Source: CAD feature listing. Evaluate the final solid. Frame: model axes, mm. Round coordinates to 2 decimals unless told otherwise and drop trailing zeros. Loops run counter-clockwise (first coordinate to the right, second up) from the corner with the lowest first, then second, coordinate; pieces in that order, holes last. Notation, with made-up numbers: M 37,12 L 46,12 A8 ccw 46,23 Z; hole C 42,72.25 d5. An arc over 180 degrees is marked long. Write each question's results on one line, items separated by ' | '. Start each with the question number.
1. Contact query for flat-ended pins moving along their axis: pin 1 Ø6 at (x, z) = (29.5, 2.5) entering from -Y; pin 2 Ø2 at (y, z) = (4, 26) entering from -X; pin 3 Ø8 at (y, z) = (4, -23) entering from -X; pin 4 Ø3 at (x, y) = (17.5, 6.5) entering from -Z. Output: stop coordinate, or through.
2. Ray query, line 1 (X direction, y = 5.5, z = -28.5); line 2 (Z direction, x = 7.5, y = 13); line 3 (X direction, y = 5.75, z = 32.5). Return the intervals inside material, ascending.
3. Draft query along X for faces 1 (the cylindrical face through (34.534, 7.395, 14.383)), 2 (the cylindrical face through (37.41, 7.4, 0.07)), 3 (the cylindrical face through (-34.59, 7.4, 14.25)). Return one class per face: released by +X, released by -X, zero draft, split by the parting line, or undercut.
4. Section B-B on z = 0. Output: boundary loops of the cut face in (x, y).
5. Section A-A on x = 0. Output: boundary loops of the cut face in (y, z), and give its area (3 significant figures).
6. Section C-C on z = -21. Output: boundary loops of the cut face in (x, y).
from build123d import *

# Parameters (mm, degrees)
SKETCH1_R           = 11
BOSS_EXTRUDE1_DEPTH = 15


with BuildPart() as part:
    # Sketch1 → Boss-Extrude1 (new body)
    with BuildSketch(Plane(origin=(0, 0, 0), x_dir=(1, 0, 0), z_dir=(0, 1, 0))):
        with BuildLine():
            ThreePointArc((40.667554182, -3.397048659), (37.40918895, 0), (40.667554182, 3.397048659))
            ThreePointArc((40.667554182, 3.397048659), (40.61268155, 4), (40.548869848, 4.602070919))
            ThreePointArc((40.548869848, 4.602070919), (36.690381874, 7.298170719), (39.223407215, 11.265621563))
            ThreePointArc((39.223407215, 11.265621563), (39.051958974, 11.846282243), (38.871915187, 12.424335493))
            ThreePointArc((38.871915187, 12.424335493), (34.561583998, 14.315876829), (36.271926705, 18.701262947))
            ThreePointArc((36.271926705, 18.701262947), (35.990491515, 19.237318503), (35.701134624, 19.769139821))
            ThreePointArc((35.701134624, 19.769139821), (31.104603832, 20.783431822), (31.926536394, 25.418225285))
            ThreePointArc((31.926536394, 25.418225285), (31.545929651, 25.889075402), (31.158379479, 26.354227193))
            ThreePointArc((31.158379479, 26.354227193), (26.452291185, 26.452291185), (26.354227193, 31.158379479))
            ThreePointArc((26.354227193, 31.158379479), (25.889075402, 31.545929651), (25.418225285, 31.926536394))
            ThreePointArc((25.418225285, 31.926536394), (20.783431822, 31.104603832), (19.769139821, 35.701134624))
            ThreePointArc((19.769139821, 35.701134624), (19.237318503, 35.990491515), (18.701262947, 36.271926705))
            ThreePointArc((18.701262947, 36.271926705), (14.315876829, 34.561583998), (12.424335493, 38.871915187))
            ThreePointArc((12.424335493, 38.871915187), (11.846282243, 39.051958974), (11.265621563, 39.223407215))
            ThreePointArc((11.265621563, 39.223407215), (7.298170719, 36.690381874), (4.602070919, 40.548869848))
            ThreePointArc((4.602070919, 40.548869848), (4, 40.61268155), (3.397048659, 40.667554182))
            ThreePointArc((3.397048659, 40.667554182), (0, 37.40918895), (-3.397048659, 40.667554182))
            ThreePointArc((-3.397048659, 40.667554182), (-4, 40.61268155), (-4.602070919, 40.548869848))
            ThreePointArc((-4.602070919, 40.548869848), (-7.298170719, 36.690381874), (-11.265621563, 39.223407215))
            ThreePointArc((-11.265621563, 39.223407215), (-11.846282243, 39.051958974), (-12.424335493, 38.871915187))
            ThreePointArc((-12.424335493, 38.871915187), (-14.315876829, 34.561583998), (-18.701262947, 36.271926705))
            ThreePointArc((-18.701262947, 36.271926705), (-19.237318503, 35.990491515), (-19.769139821, 35.701134624))
            ThreePointArc((-19.769139821, 35.701134624), (-20.783431822, 31.104603832), (-25.418225285, 31.926536394))
            ThreePointArc((-25.418225285, 31.926536394), (-25.889075402, 31.545929651), (-26.354227193, 31.158379479))
            ThreePointArc((-26.354227193, 31.158379479), (-26.452291185, 26.452291185), (-31.158379479, 26.354227193))
            ThreePointArc((-31.158379479, 26.354227193), (-31.545929651, 25.889075402), (-31.926536394, 25.418225285))
            ThreePointArc((-31.926536394, 25.418225285), (-31.104603832, 20.783431822), (-35.701134624, 19.769139821))
            ThreePointArc((-35.701134624, 19.769139821), (-35.990491515, 19.237318503), (-36.271926705, 18.701262947))
            ThreePointArc((-36.271926705, 18.701262947), (-34.561583998, 14.315876829), (-38.871915187, 12.424335493))
            ThreePointArc((-38.871915187, 12.424335493), (-39.051958974, 11.846282243), (-39.223407215, 11.265621563))
            ThreePointArc((-39.223407215, 11.265621563), (-36.690381874, 7.298170719), (-40.548869848, 4.602070919))
            ThreePointArc((-40.548869848, 4.602070919), (-40.61268155, 4), (-40.667554182, 3.397048659))
            ThreePointArc((-40.667554182, 3.397048659), (-37.40918895, 0), (-40.667554182, -3.397048659))
            ThreePointArc((-40.667554182, -3.397048659), (-40.61268155, -4), (-40.548869848, -4.602070919))
            ThreePointArc((-40.548869848, -4.602070919), (-36.690381874, -7.298170719), (-39.223407215, -11.265621563))
            ThreePointArc((-39.223407215, -11.265621563), (-39.051958974, -11.846282243), (-38.871915187, -12.424335493))
            ThreePointArc((-38.871915187, -12.424335493), (-34.561583998, -14.315876829), (-36.271926705, -18.701262947))
            ThreePointArc((-36.271926705, -18.701262947), (-35.990491515, -19.237318503), (-35.701134624, -19.769139821))
            ThreePointArc((-35.701134624, -19.769139821), (-31.104603832, -20.783431822), (-31.926536394, -25.418225285))
            ThreePointArc((-31.926536394, -25.418225285), (-31.545929651, -25.889075402), (-31.158379479, -26.354227193))
            ThreePointArc((-31.158379479, -26.354227193), (-26.452291185, -26.452291185), (-26.354227193, -31.158379479))
            ThreePointArc((-26.354227193, -31.158379479), (-25.889075402, -31.545929651), (-25.418225285, -31.926536394))
            ThreePointArc((-25.418225285, -31.926536394), (-20.783431822, -31.104603832), (-19.769139821, -35.701134624))
            ThreePointArc((-19.769139821, -35.701134624), (-19.237318503, -35.990491515), (-18.701262947, -36.271926705))
            ThreePointArc((-18.701262947, -36.271926705), (-14.315876829, -34.561583998), (-12.424335493, -38.871915187))
            ThreePointArc((-12.424335493, -38.871915187), (-11.846282243, -39.051958974), (-11.265621563, -39.223407215))
            ThreePointArc((-11.265621563, -39.223407215), (-7.298170719, -36.690381874), (-4.602070919, -40.548869848))
            ThreePointArc((-4.602070919, -40.548869848), (-4, -40.61268155), (-3.397048659, -40.667554182))
            ThreePointArc((-3.397048659, -40.667554182), (0, -37.40918895), (3.397048659, -40.667554182))
            ThreePointArc((3.397048659, -40.667554182), (4, -40.61268155), (4.602070919, -40.548869848))
            ThreePointArc((4.602070919, -40.548869848), (7.298170719, -36.690381874), (11.265621563, -39.223407215))
            ThreePointArc((11.265621563, -39.223407215), (11.846282243, -39.051958974), (12.424335493, -38.871915187))
            ThreePointArc((12.424335493, -38.871915187), (14.315876829, -34.561583998), (18.701262947, -36.271926705))
            ThreePointArc((18.701262947, -36.271926705), (19.237318503, -35.990491515), (19.769139821, -35.701134624))
            ThreePointArc((19.769139821, -35.701134624), (20.783431822, -31.104603832), (25.418225285, -31.926536394))
            ThreePointArc((25.418225285, -31.926536394), (25.889075402, -31.545929651), (26.354227193, -31.158379479))
            ThreePointArc((26.354227193, -31.158379479), (26.452291185, -26.452291185), (31.158379479, -26.354227193))
            ThreePointArc((31.158379479, -26.354227193), (31.545929651, -25.889075402), (31.926536394, -25.418225285))
            ThreePointArc((31.926536394, -25.418225285), (31.104603832, -20.783431822), (35.701134624, -19.769139821))
            ThreePointArc((35.701134624, -19.769139821), (35.990491515, -19.237318503), (36.271926705, -18.701262947))
            ThreePointArc((36.271926705, -18.701262947), (34.561583998, -14.315876829), (38.871915187, -12.424335493))
            ThreePointArc((38.871915187, -12.424335493), (39.051958974, -11.846282243), (39.223407215, -11.265621563))
            ThreePointArc((39.223407215, -11.265621563), (36.690381874, -7.298170719), (40.548869848, -4.602070919))
            ThreePointArc((40.548869848, -4.602070919), (40.61268155, -4), (40.667554182, -3.397048659))
        make_face()
        with Locations(Location((0, 0, 0), (0, 0, 270))):
            Circle(SKETCH1_R, mode=Mode.SUBTRACT)
    extrude(amount=BOSS_EXTRUDE1_DEPTH)


solid = part.part
Taken from the geometry:
1) pin 1: y = 0 | pin 2: x = -31.93 | pin 3: x = -36.12 | pin 4: z = -36.27
2) line 1: -25.48 to 25.48 | line 2: -36.66 to -8.05, 8.05 to 36.66 | line 3: -19.59 to 19.59
3) face 1: undercut | face 2: released by +X | face 3: undercut
4) outline: M -37.41,0 L -11,0 L -11,15 L -37.41,15 Z; M 11,0 L 37.41,0 L 37.41,15 L 11,15 Z
5) outline: M 0,-37.41 L 15,-37.41 L 15,-11 L 0,-11 Z; M 0,11 L 15,11 L 15,37.41 L 0,37.41 Z | area: 792 mm^2
6) outline: M -30.97,0 L 30.97,0 L 30.97,15 L -30.97,15 Z
